```python
from build123d import *

# Parameters (mm, degrees)
SKETCH_1_W          = 10
SKETCH_1_H          = 10
SKETCH_1_W_2        = 8
SKETCH_1_H_2        = 8
EXTRUDE_1_DEPTH     = 125
SKETCH_2_R          = 1.6
CUT_EXTRUDE_1_DEPTH = 126.49900398
SKETCH_3_R          = 1.6
CUT_EXTRUDE_2_DEPTH = 126.49900398
SKETCH_4_R          = 1.6
CUT_EXTRUDE_3_DEPTH = 126.49900398


with BuildPart() as part:
    # ｽｹｯﾁ1 → ﾎﾞｽ - 押し出し1 (new body)
    with BuildSketch(Plane.XY):
        Rectangle(SKETCH_1_W, SKETCH_1_H)
        Rectangle(SKETCH_1_W_2, SKETCH_1_H_2, mode=Mode.SUBTRACT)
    extrude(amount=EXTRUDE_1_DEPTH)

    # ｽｹｯﾁ2 → ｶｯﾄ - 押し出し1 (cut, through all)
    with BuildSketch(Plane.XZ.offset(5)):
        with Locations(Location((0, 5, 0), (0, 0, 270))):
            Circle(SKETCH_2_R)
        with Locations(Location((0, 80, 0), (0, 0, 270))):
            Circle(SKETCH_2_R)
        with Locations(Location((0, 120, 0), (0, 0, 270))):
            Circle(SKETCH_2_R)
    extrude(amount=-CUT_EXTRUDE_1_DEPTH, mode=Mode.SUBTRACT)

    # ｽｹｯﾁ3 → ｶｯﾄ - 押し出し2 (cut, through all)
    with BuildSketch(Plane(origin=(5, 0, 0), x_dir=(0, 0, -1), z_dir=(1, 0, 0))):
        with Locations(Location((-15, 0, 0), (0, 0, 90))):
            Circle(SKETCH_3_R)
    extrude(amount=-CUT_EXTRUDE_2_DEPTH, mode=Mode.SUBTRACT)

    # ｽｹｯﾁ4 → ｶｯﾄ - 押し出し3 (cut, through all)
    with BuildSketch(Plane(origin=(5, 0, 0), x_dir=(0, 0, -1), z_dir=(1, 0, 0))):
        with Locations(Location((-47.989898732, 0, 0), (0, 0, 90))):
            Circle(SKETCH_4_R)
    extrude(amount=-CUT_EXTRUDE_3_DEPTH, mode=Mode.SUBTRACT)


solid = part.part
```
Geometry: final body of the model. Coordinates: model frame, mm. A direction names the side the tool comes from. Coordinates: 2 decimals unless noted, no trailing zeros. Write each loop counter-clockwise with the first axis right and the second up, starting at its lowest first coordinate (ties: lowest second). Pieces come first, ordered by that corner, then holes. Notation, with made-up numbers: M -22,87 L 31,87 A13 ccw 31,100 Z; hole C 68.5,43 d8. An arc over 180 degrees is marked long. Use CSV: the item, a comma, the result in double quotes. Start each with the question number.
1. Reachability of faces 4 (the face through (-0.97, -4.51, 6.27)), 5 (the face through (4, 0, 62)) from +Z, -Z, +X, -X, +Y, -Y: full face, straight path, thin tool, end or side. Return the list, or none.
2. Cut plane C-C on z = 5. Return the cut outline in (x, y).
3. Ray query, probe 1 along Z at (x, y) = (4.6, 0); probe 2 along X at (y, z) = (-1.5, 103). Return the intervals inside material, ascending.
4. Cut plane B-B on z = 95. Return the cut outline in (x, y), plus the area to 3 significant figures.
5. Mould query, pull axis Z, two halves, no side actions, for faces 1 (the face through (0.481, 4.493, 118.474)), 2 (the face through (-4.5, 0.1, 0)), 3 (the face through (0, -4, 62)). Classes: pulls with the +Z half, pulls with the -Z half, needs draft (parallel to the pull), parting line crosses it, or undercut.
6. Cut plane A-A on y = -2.75. Return the cut outline in (x, z).
7. First-contact query: P1, Ø4, axis at x = 0, z = 5, coming from the -Y side; P2, Ø2.5, axis at y = 0, z = 47.99, coming from the +X side. Flat tips, straight axial feed; report the tip coordinate or a pass-through.
Entries:
1,face 4,"+Y, -Y"
1,face 5,"+Z, -Z"
2,outline,"M -5,-5 L -1.6,-5 L -1.6,-4 L -4,-4 L -4,4 L -1.6,4 L -1.6,5 L -5,5 Z; M 1.6,-5 L 5,-5 L 5,5 L 1.6,5 L 1.6,4 L 4,4 L 4,-4 L 1.6,-4 Z"
3,probe 1,"0 to 13.4, 16.6 to 46.39, 49.59 to 125"
3,probe 2,"-5 to -4, 4 to 5"
4,outline,"M -5,-5 L 5,-5 L 5,5 L -5,5 Z; hole M -4,-4 L 4,-4 L 4,4 L -4,4 Z"
4,area,"36.0 mm²"
5,face 1,"undercut"
5,face 2,"pulls with the -Z half"
5,face 3,"needs draft"
6,outline,"M -5,0 L -4,0 L -4,125 L -5,125 Z; M 4,0 L 5,0 L 5,125 L 4,125 Z"
7,P1,"y = -5"
7,P2,"through"
